from build123d import *

# Parameters (mm, degrees)
F0_W     = 197.526522
F0_H     = 96.156877
F0_R     = 27.452888
F1_DEPTH = 25.4


with BuildPart() as f1:
    # F0 (on Front) → F1 (new body)
    with BuildSketch(Plane.XZ):
        with Locations((35.741519, 10.025931)):
            Rectangle(F0_W, F0_H)
        with Locations((11.08718, 19.393688)):
            Circle(F0_R, mode=Mode.SUBTRACT)
        Polygon((113.338566, 26.044908), (105.036274, -10.088419), (68.105889, -13.358281), (53.583948, 20.754159), (81.53928, 45.106669), align=None, mode=Mode.SUBTRACT)
    extrude(amount=F1_DEPTH)


solid = f1.part
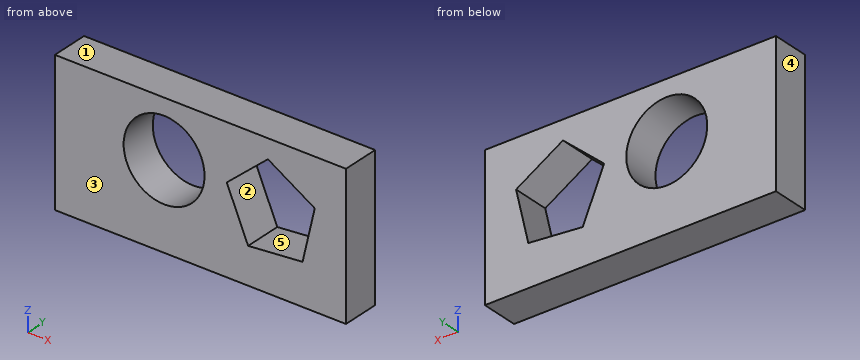
Can you work these out from the model? Positions are in its coordinate system, mm. Face numbers are marked on the shaded views. A direction names the side the tool comes from. Coordinates: 2 decimals unless noted, no trailing zeros. Write each loop counter-clockwise with the first axis right and the second up, starting at its lowest first coordinate (ties: lowest second). Pieces come first, ordered by that corner, then holes.
Q1. If we mould it in two halves opening along X, with no side actions, what happens to the marked faces 3, 4 and 5? For each: +X half, -X half, draft (parallel to the pull), parting line (faces both ways), or undercut.
Results found:
face 3: draft
face 4: -X half
face 5: undercut
Q2. Imagine slicing it at A-A, the plane x = -8. List the corners of the cut face in (y, z) for me, plus the area to 3 significant figures.
Results found:
outline: (-25.4, -38.05) - (0, -38.05) - (0, -0.34) - (-25.4, -0.34) - close; (-25.4, 39.13) - (0, 39.13) - (0, 58.1) - (-25.4, 58.1) - close
area: 1,440 mm2
Q3. Imagine slicing it at D-D, the plane x = 93. List the corners of the cut face in (y, z) for me, plus the area to 3 significant figures.
Results found:
outline: (-25.4, -38.05) - (0, -38.05) - (0, -11.15) - (-25.4, -11.15) - close; (-25.4, 38.24) - (0, 38.24) - (0, 58.1) - (-25.4, 58.1) - close
area: 1,190 mm2
Q4. Imagine slicing it at C-C, the plane y = -4.75. List the corners of the cut face in (x, z) for me, plus the area to 3 significant figures.
Results found:
outline: (-63.02, -38.05) - (134.5, -38.05) - (134.5, 58.1) - (-63.02, 58.1) - close; hole circle Ø54.91 at (11.09, 19.39); hole (53.58, 20.75) - (68.11, -13.36) - (105.04, -10.09) - (113.34, 26.04) - (81.54, 45.11) - close
area: 14,300 mm2
Q5. Imagine slicing it at B-B, the plane z = 17.5. List the corners of the cut face in (x, y) for me, plus the area to 3 significant figures.
Results found:
outline: (-63.02, -25.4) - (-16.3, -25.4) - (-16.3, 0) - (-63.02, 0) - close; (38.47, -25.4) - (54.97, -25.4) - (54.97, 0) - (38.47, 0) - close; (111.38, -25.4) - (134.5, -25.4) - (134.5, 0) - (111.38, 0) - close
area: 2,190 mm2
Q6. Which directions (+Z, -Z, +X, -X, +Y, -Y) give clear straight access to the entire face, cutting with the end or side of a thin tool? Please do the marked faces 1 and 2.
Results found:
face 1: +Z, +X, -X, +Y, -Y
face 2: +Y, -Y
Q7. Please list where these lines run through material, in increasing order: L1, parallel to X at y = -6.5, z = 44.5; L2, parallel to X at y = -7, z = 36; L3, parallel to Z at x = -12.5, y = -20.5.
Results found:
L1: x = -63.02 to -0.02, 22.19 to 80.84, 82.55 to 134.5
L2: x = -63.02 to -10.77, 32.95 to 71.09, 96.73 to 134.5
L3: z = -38.05 to 5.35, 33.44 to 58.1
